Check sheet for the modelled part. Datum: model origin and axes. Units: mm. Face numbers are marked on the shaded views. A direction names the side the tool comes from. Round coordinates to 2 decimals unless told otherwise and drop trailing zeros. Order: outer loops, then holes, each group sorted by start corner. A loop starts at its lowest first (then second) coordinate and runs counter-clockwise, first axis right, second up.
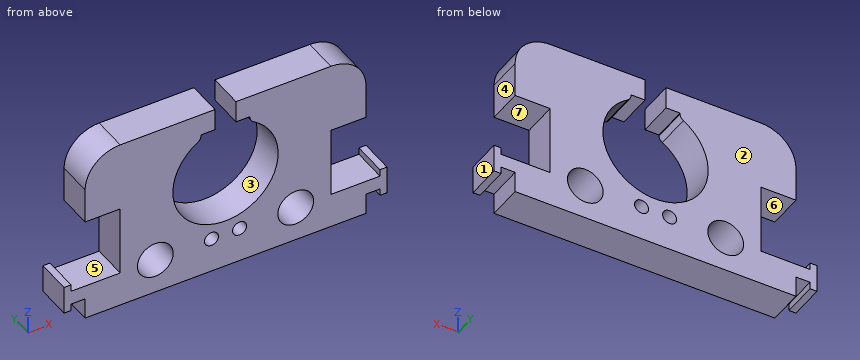
from build123d import *

# Parameters (mm, degrees)
SKETCH_1_R      = 2.55
SKETCH_1_R_2    = 1
EXTRUDE_1_DEPTH = 5


with BuildPart() as part:
    # 草图1 → 凸台-拉伸1 (new body)
    with BuildSketch(Plane(origin=(0, 0, 0), x_dir=(1, 0, 0), z_dir=(0, 1, 0))):
        with BuildLine():
            Line((35, 20), (37, 20))
            Line((37, 20), (37, 19))
            Line((37, 19), (38, 19))
            Line((38, 19), (38, 23))
            Line((38, 23), (37, 23))
            Line((37, 23), (37, 22))
            Line((37, 22), (35, 22))
            Line((35, 22), (35, 25))
            Line((35, 25), (30, 25))
            Line((30, 25), (20, 25))
            Line((20, 25), (10, 25))
            Line((10, 25), (0, 25))
            Line((0, 25), (-5, 25))
            Line((-5, 25), (-5, 22))
            Line((-5, 22), (-7, 22))
            Line((-7, 22), (-7, 23))
            Line((-7, 23), (-8, 23))
            Line((-8, 23), (-8, 19))
            Line((-8, 19), (-7, 19))
            Line((-7, 19), (-7, 20))
            Line((-7, 20), (-5, 20))
            Line((-5, 20), (0, 20))
            Line((0, 20), (0, 10))
            Line((0, 10), (-5, 10))
            Line((-5, 10), (-5, 5))
            ThreePointArc((-5, 5), (-3.535533906, 1.464466094), (0, 0))
            Line((0, 0), (5, 0))
            Line((5, 0), (13.5, 0))
            Line((13.5, 0), (13.5, 3.151530772))
            Line((13.5, 3.151530772), (11.5, 3.151530772))
            Line((11.5, 3.151530772), (11.5, 3.288897449))
            ThreePointArc((11.5, 3.288897449), (11.374474632, 3.773968699), (11.029411765, 4.137262455))
            ThreePointArc((11.029411765, 4.137262455), (15, 18), (18.970588235, 4.137262455))
            ThreePointArc((18.970588235, 4.137262455), (18.625525368, 3.773968699), (18.5, 3.288897449))
            Line((18.5, 3.288897449), (18.5, 3.151530772))
            Line((18.5, 3.151530772), (16.5, 3.151530772))
            Line((16.5, 3.151530772), (16.5, 0))
            Line((16.5, 0), (25, 0))
            Line((25, 0), (30, 0))
            ThreePointArc((30, 0), (33.535533906, 1.464466094), (35, 5))
            Line((35, 5), (35, 10))
            Line((35, 10), (30, 10))
            Line((30, 10), (30, 20))
            Line((30, 20), (35, 20))
        make_face()
        with Locations(Location((5, 20, 0), (0, 0, 270))):
            Circle(SKETCH_1_R, mode=Mode.SUBTRACT)
        with Locations(Location((25, 20, 0), (0, 0, 270))):
            Circle(SKETCH_1_R, mode=Mode.SUBTRACT)
        with Locations(Location((13, 20, 0), (0, 0, 270))):
            Circle(SKETCH_1_R_2, mode=Mode.SUBTRACT)
        with Locations(Location((17, 20, 0), (0, 0, 270))):
            Circle(SKETCH_1_R_2, mode=Mode.SUBTRACT)
    extrude(amount=EXTRUDE_1_DEPTH)


solid = part.part
1) Draft check along X on the marked faces 1, 2 and 3. Enter one of: pulls with the +X half, pulls with the -X half, needs draft (parallel to the pull), parting line crosses it, or undercut.
2) Sectioned sample at B-B on z = -8.5. Record the cut outline in (x, y).
3) Sectioned sample at D-D on x = 17. Record the cut outline in (y, z), and give its area (3 significant figures).
4) Gauge pin test, flat ends, axial feed: pin 1 (3 mm diameter, centred on y = 2.5, z = -17, fed in from -X); pin 2 (1.1 mm diameter, centred on x = -7.5, y = 3.5, fed in from -Z); pin 3 (2.5 mm diameter, centred on y = 2.5, z = -1, fed in from -X). Record the tip position at first contact, or that the pin passes through.
5) Sectioned sample at C-C on y = 4.3. Count the separate pieces of the cut face and the enclosed holes in it, and give its area (3 significant figures).
6) Set-up check for the marked faces 4, 5, 6 and 7: record each of +Z, -Z, +X, -X, +Y, -Y from which the full face is reachable in a straight line by a thin tool's end or side.
7) Sectioned sample at A-A on x = 5. Record the cut outline in (y, z), and give its area (3 significant figures).
8) Scan lines: line 1 (X direction, y = 2.9, z = -21.25); line 2 (X direction, y = 2.75, z = -10.5); line 3 (X direction, y = 0.25, z = -20.75). Record each from-to range of solid material in increasing order.
Values found:
1. face 1: pulls with the +X half
1. face 2: needs draft
1. face 3: undercut
2. outline: (-5, 0) - (7.77, 0) - (7.77, 5) - (-5, 5) - close; (22.23, 0) - (35, 0) - (35, 5) - (22.23, 5) - close
3. outline: (0, -25) - (5, -25) - (5, -21) - (0, -21) - close; (0, -19) - (5, -19) - (5, -17.73) - (0, -17.73) - close; (0, -3.15) - (5, -3.15) - (5, 0) - (0, 0) - close
3. area: 42.1 mm2
4. pin 1: stops at x = 0
4. pin 2: stops at z = -23
4. pin 3: stops at x = -4.18
5. separate pieces: 1
5. enclosed holes: 4
5. area: 671 mm2
6. face 4: +Z, +X, +Y, -Y
6. face 5: +Y, -Y
6. face 6: -X, +Y, -Y
6. face 7: +X, +Y, -Y
7. outline: (0, -25) - (5, -25) - (5, -22.55) - (0, -22.55) - close; (0, -17.45) - (5, -17.45) - (5, 0) - (0, 0) - close
7. area: 99.5 mm2
8. line 1: x = -8 to 2.78, 7.22 to 22.78, 27.22 to 38
8. line 2: x = 0 to 7.5, 22.5 to 30
8. line 3: x = -8 to 2.56, 7.44 to 12.34, 13.66 to 16.34, 17.66 to 22.56, 27.44 to 38
